Model file for the job. Use its own axes, mm. A direction names the side the tool comes from. Coordinates: 2 decimals unless noted, no trailing zeros. Write each loop counter-clockwise with the first axis right and the second up, starting at its lowest first coordinate (ties: lowest second). Pieces come first, ordered by that corner, then holes. Notation, with made-up numbers: M 48.25,56.25 L 62.25,56.25 A14 cw 62.25,76.25 Z; hole C 7.25,51 d3. An arc over 180 degrees is marked long. Use CSV: the item, a comma, the result in double quotes. Start each with the question number.
from build123d import *

# Parameters (mm, degrees)
SKETCH1_W               = 100
SKETCH1_H               = 80
BOSS_EXTRUDE1_DEPTH     = 40
CUT_EXTRUDE1_REACH      = 77.498
SKETCH2_R               = 7.5
SKETCH2_R_2             = 10.5
CUT_EXTRUDE2_REACH      = 77.498
SKETCH3_W               = 100
SKETCH3_H               = 20
CUT_EXTRUDE3_DEPTH      = 50
CUT_EXTRUDE3_DEPTH_BACK = 25
SKETCH4_R               = 3
CUT_EXTRUDE4_REACH      = 77.498
SKETCH5_W               = 50
SKETCH5_H               = 25
FILLET1_R               = 10
FILLET2_R               = 10
FILLET3_R               = 10
FILLET4_R               = 10
SKETCH6_W               = 50
SKETCH6_H               = 40
SKETCH6_W_2             = 40
SKETCH6_H_2             = 30
BOSS_EXTRUDE2_DEPTH     = 10


with BuildPart() as part:
    # Sketch1 → Boss-Extrude1 (new body)
    with BuildSketch(Plane.XY):
        Rectangle(SKETCH1_W, SKETCH1_H)
    extrude(amount=BOSS_EXTRUDE1_DEPTH)

    # Sketch2 → Cut-Extrude1 (cut, up to next)
    with BuildSketch(Plane.XY.offset(40), mode=Mode.PRIVATE) as cut_extrude1_sk1:
        Circle(SKETCH2_R)
    cut_extrude1_tool1 = extrude(cut_extrude1_sk1.sketch, amount=-CUT_EXTRUDE1_REACH, mode=Mode.PRIVATE) & part.part
    # Sketch2 → Cut-Extrude1 (cut, up to next)
    with BuildSketch(Plane.XY.offset(40), mode=Mode.PRIVATE) as cut_extrude1_sk2:
        with Locations((-35, 0)):
            Circle(SKETCH2_R_2)
    cut_extrude1_tool2 = extrude(cut_extrude1_sk2.sketch, amount=-CUT_EXTRUDE1_REACH, mode=Mode.PRIVATE) & part.part
    # Sketch2 → Cut-Extrude1 (cut, up to next)
    with BuildSketch(Plane.XY.offset(40), mode=Mode.PRIVATE) as cut_extrude1_sk3:
        with Locations((35, 0)):
            Circle(SKETCH2_R_2)
    cut_extrude1_tool3 = extrude(cut_extrude1_sk3.sketch, amount=-CUT_EXTRUDE1_REACH, mode=Mode.PRIVATE) & part.part
    add(cut_extrude1_tool1.solids().sort_by_distance((0, 0, 40))[0], mode=Mode.SUBTRACT)
    add(cut_extrude1_tool2.solids().sort_by_distance((-35, 0, 40))[0], mode=Mode.SUBTRACT)
    add(cut_extrude1_tool3.solids().sort_by_distance((35, 0, 40))[0], mode=Mode.SUBTRACT)

    # Sketch3 → Cut-Extrude2 (cut, up to next)
    with BuildSketch(Plane.XY.offset(40), mode=Mode.PRIVATE) as cut_extrude2_sk1:
        with Locations((0, 30)):
            Rectangle(SKETCH3_W, SKETCH3_H)
    cut_extrude2_tool1 = extrude(cut_extrude2_sk1.sketch, amount=-CUT_EXTRUDE2_REACH, mode=Mode.PRIVATE) & part.part
    add(cut_extrude2_tool1.solids().sort_by_distance((0, 30, 40))[0], mode=Mode.SUBTRACT)

    # Sketch4 → Cut-Extrude3 (cut, two sides: drawn at the far end of the back side and taken through both)
    with BuildSketch(Plane.XZ.offset(40).offset(-CUT_EXTRUDE3_DEPTH_BACK)):
        with Locations(Location((16, 20, 0), (0, 0, 180))):
            Circle(SKETCH4_R)
        with Locations(Location((36, 20, 0), (0, 0, 180))):
            Circle(SKETCH4_R)
    extrude(amount=CUT_EXTRUDE3_DEPTH + CUT_EXTRUDE3_DEPTH_BACK, mode=Mode.SUBTRACT)

    # Sketch5 → Cut-Extrude4 (cut, up to next)
    with BuildSketch(Plane(origin=(0, 0, 0), x_dir=(-1, 0, 0), z_dir=(0, 0, -1)), mode=Mode.PRIVATE) as cut_extrude4_sk1:
        with Locations((25, -27.5)):
            Rectangle(SKETCH5_W, SKETCH5_H)
    cut_extrude4_tool1 = extrude(cut_extrude4_sk1.sketch, amount=-CUT_EXTRUDE4_REACH, mode=Mode.PRIVATE) & part.part
    add(cut_extrude4_tool1.solids().sort_by_distance((-25, -27.5, 0))[0], mode=Mode.SUBTRACT)

    # Fillet1
    fillet1_edges = [part.edges().sort_by_distance(p)[0] for p in [
        (0, -15, 20),
    ]]
    fillet(fillet1_edges, radius=FILLET1_R)

    # Fillet2
    fillet2_edges = [part.edges().sort_by_distance(p)[0] for p in [
        (-50, -15, 20),
    ]]
    fillet(fillet2_edges, radius=FILLET2_R)

    # Fillet3
    fillet3_edges = [part.edges().sort_by_distance(p)[0] for p in [
        (-50, 20, 20),
    ]]
    fillet(fillet3_edges, radius=FILLET3_R)

    # Fillet4
    fillet4_edges = [part.edges().sort_by_distance(p)[0] for p in [
        (50, 20, 20),
    ]]
    fillet(fillet4_edges, radius=FILLET4_R)

    # Sketch6 → Boss-Extrude2 (add)
    with BuildSketch(Plane.XZ.offset(40)):
        with Locations((25, 20)):
            Rectangle(SKETCH6_W, SKETCH6_H)
        with Locations((25, 20)):
            Rectangle(SKETCH6_W_2, SKETCH6_H_2, mode=Mode.SUBTRACT)
    extrude(amount=BOSS_EXTRUDE2_DEPTH)


solid = part.part
1) Band-saw the part on C-C on y = 0. List the corners of the cut face in (x, z), then the cut area to 3 significant figures.
2) Band-saw the part on A-A on x = -35. List the corners of the cut face in (y, z), then the cut area to 3 significant figures.
3) Band-saw the part on D-D on x = 16. List the corners of the cut face in (y, z).
4) Tool access for faces 5 (the face through (24.51, 0.46, 20.28)), 6 (the face through (0, -37, 20)), 7 (the face through (45, -45, 20)): list every direction of +Z, -Z, +X, -X, +Y, -Y with a clear straight run to the whole face (end or side of a thin tool).
5) Wall check: L1, parallel to X at y = -28.5, z = 20; L2, parallel to X at y = -44, z = 17.5; L3, parallel to Y at x = 34.5, z = 18.5. Give the ranges that are in metal, low to high. Write a range as [from, to].
6) Band-saw the part on B-B on z = 26. List the corners of the cut face in (x, y), then the cut area to 3 significant figures.
7) Drop flat-ended pins along their axis: P1, Ø24, axis at x = 33.5, z = 26.5, coming from the -Y side; P2, Ø6, axis at x = 25.5, z = 18, coming from the -Y side; P3, Ø5, axis at x = 16, z = 20, coming from the -Y side; P4, Ø24, axis at x = -20, z = 23, coming from the -Y side. Give the stop position or say it passes through.
8) Two-plate mould, pull along X, no slides. Class faces 1 (the face through (50, -20, 20)), 2 (the face through (-3.01, -17.85, 20.28)), 3 (the face through (10, -7, 40)), 4 (the face through (39, -27, 20)): pulls with the +X half, pulls with the -X half, needs draft (parallel to the pull), parting line crosses it, or undercut.
Findings below:
1,outline,"M -50,0 L -45.5,0 L -45.5,40 L -50,40 Z; M -24.5,0 L -7.5,0 L -7.5,40 L -24.5,40 Z; M 7.5,0 L 24.5,0 L 24.5,40 L 7.5,40 Z; M 45.5,0 L 50,0 L 50,40 L 45.5,40 Z"
1,area,"1,720 mm2"
2,outline,"M -15,0 L -10.5,0 L -10.5,40 L -15,40 Z; M 10.5,0 L 20,0 L 20,40 L 10.5,40 Z"
2,area,"560 mm2"
3,outline,"M -50,0 L 20,0 L 20,40 L -50,40 L -50,35 L -40,35 L -40,23 L -15,23 L -15,17 L -40,17 L -40,5 L -50,5 Z"
4,face 5,"+Z, -Z"
4,face 6,"+Z, -Z, -X, -Y"
4,face 7,"-Y"
5,L1,"x = [0, 13], [19, 33], [39, 50]"
5,L2,"x = [0, 5], [45, 50]"
5,L3,"y = [-15, -10.49], [10.49, 20]"
6,outline,"M -50,-5 A10 ccw -40,-15 L -10,-15 A10 cw 0,-25 L 0,-50 L 5,-50 L 5,-40 L 45,-40 L 45,-50 L 50,-50 L 50,10 A10 ccw 40,20 L -40,20 A10 ccw -50,10 Z; hole C -35,0 d21; hole C 0,0 d15; hole C 35,0 d21"
6,area,"3,940 mm2"
7,P1,"stops at y = -50"
7,P2,"stops at y = -40"
7,P3,"stops at y = -15"
7,P4,"stops at y = -15.2"
8,face 1,"pulls with the +X half"
8,face 2,"pulls with the -X half"
8,face 3,"needs draft"
8,face 4,"undercut"
